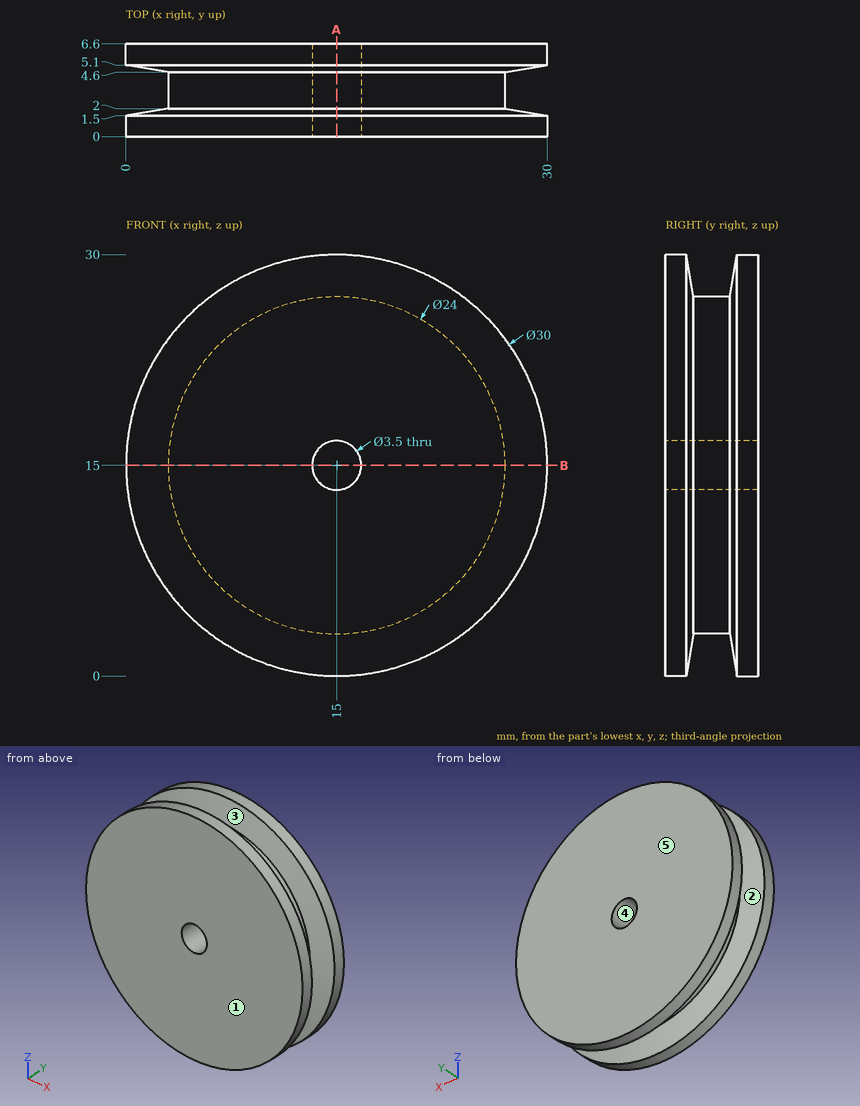
Source: three-view drawing plus pictorial views. Frame: mm from the lowest corner of the part. A direction names the side the tool comes from. Give positions to 0.01 mm unless a question says otherwise; leave off trailing zeros. Write each loop counter-clockwise with the first axis right and the second up, starting at its lowest first coordinate (ties: lowest second). Pieces come first, ordered by that corner, then holes. Notation, with made-up numbers: (-12, 52) -> (19, 52) arc R10 cw to (19, 58) -> close; hole circle Ø6 at (67, -1.75). An arc over 180 degrees is marked (long way). Write item = value, one per line.
Q1. Cut plane A-A on x = 15. Return loops of the section in (y, z), then the cut area to 3 significant figures.
Here are the results:
outline = (0, 0) -> (1.5, 0) -> (2, 3) -> (4.6, 3) -> (5.1, 0) -> (6.6, 0) -> (6.6, 13.25) -> (0, 13.25) -> close; (0, 16.75) -> (6.6, 16.75) -> (6.6, 30) -> (5.1, 30) -> (4.6, 27) -> (2, 27) -> (1.5, 30) -> (0, 30) -> close
area = 156 mm²
Q2. Cut plane B-B on z = 15. Return loops of the section in (x, y), then the cut area to 3 significant figures.
Here are the results:
outline = (0, 0) -> (13.25, 0) -> (13.25, 6.6) -> (0, 6.6) -> (0, 5.1) -> (3, 4.6) -> (3, 2) -> (0, 1.5) -> close; (16.75, 0) -> (30, 0) -> (30, 1.5) -> (27, 2) -> (27, 4.6) -> (30, 5.1) -> (30, 6.6) -> (16.75, 6.6) -> close
area = 156 mm²
Q3. First-contact query: pin 1 (1.5 mm diameter, centred on x = 10, y = 3.5, fed in from -Z); pin 2 (2 mm diameter, centred on x = 16, y = 5, fed in from +Z); pin 3 (3 mm diameter, centred on x = 24, y = 1.5, fed in from -Z). Flat tips, straight axial feed; report the tip coordinate or a pass-through.
Here are the results:
pin_1 = 3.78
pin_2 = 30
pin_3 = 2.01
Q4. Line query: line 1 (Y direction, x = 3, z = 17); line 2 (X direction, y = 3.25, z = 15.75); line 3 (Y direction, x = 25, z = 24.5). Output: solid intervals per line, ascending. Write a range as from..to.
Here are the results:
line_1 = 0..1.97, 4.63..6.6
line_2 = 3.02..13.42, 16.58..26.98
line_3 = 0..1.7, 4.9..6.6
Q5. Mould query, pull axis Y, two halves, no side actions, for the marked faces 3, 4 and 5. Classes: +Y half, -Y half, draft (parallel to the pull), parting line (faces both ways), or undercut.
Here are the results:
face_3 = undercut
face_4 = draft
face_5 = +Y half
Q6. Reachability of the marked faces 1 and 2 from +Z, -Z, +X, -X, +Y, -Y: full face, straight path, thin tool, end or side. Return the list, or none.
Here are the results:
face_1 = +Z, -Z, +X, -X, -Y
face_2 = none
